```python
from build123d import *

# Parameters (mm, degrees)
SKETCH1_R           = 2
BOSS_EXTRUDE1_DEPTH = 6.35


with BuildPart() as part:
    # Sketch1 → Boss-Extrude1 (new body)
    with BuildSketch(Plane(origin=(0, 0, 0), x_dir=(1, 0, 0), z_dir=(0, 1, 0))):
        with BuildLine():
            Line((12.7, 0), (12.7, 6.35))
            ThreePointArc((12.7, 6.35), (14.559871939, 10.840128061), (19.05, 12.7))
            Line((19.05, 12.7), (39.168815004, 12.7))
            ThreePointArc((39.168815004, 12.7), (45.084999997, 15.87476101), (39.169071524, 19.05))
            Line((39.169071524, 19.05), (12.7, 19.05))
            Line((12.7, 19.05), (10.16, 19.05))
            ThreePointArc((10.16, 19.05), (2.975795103, 16.074204897), (0, 8.89))
            Line((0, 8.89), (0, 0))
            Line((0, 0), (12.7, 0))
        make_face()
        with Locations((41.275, 15.874914922)):
            Circle(SKETCH1_R, mode=Mode.SUBTRACT)
    extrude(amount=BOSS_EXTRUDE1_DEPTH)


solid = part.part
```
The model under review builds one solid part; all positions refer to its coordinate system, in mm. A direction names the side the tool comes from. Round coordinates to 2 decimals unless told otherwise and drop trailing zeros. Loops run counter-clockwise (first coordinate to the right, second up) from the corner with the lowest first, then second, coordinate; pieces in that order, holes last. Notation, with made-up numbers: (7, 53.5) - (56, 53.5) arc R30 cw to (56, 87.5) - close; hole circle Ø4 at (68, 11). An arc over 180 degrees is marked (long way). Use a Markdown table: item, result. Add a question column.
Q1. The part is to be moulded in two halves that separate along X. For faces 1 (the face through (17, 0, -14)), 2 (the face through (14.51, 3.13, -10.79)), 3 (the face through (12.7, 3, -3)), say which applies: pulls with the +X half, pulls with the -X half, needs draft (parallel to the pull), parting line crosses it, or undercut.
Q2. Machinability: for faces 4 (the face through (25, 3, -19.05)), 5 (the face through (39.801, 3.131, -17.227)), 6 (the face through (29, 3, -12.7)), which of the approach directions +Z, -Z, +X, -X, +Y, -Y give a long, thin tool a straight path to every point of the face, cutting with its end or side? Answer none if there is none.
Q3. Add section C-C (y = 2.75). State the section outline as (x, z) points (3 decimals), plus the area to 3 significant figures.
Q4. Add section D-D (x = 26.5). State the section outline as (y, z) points, plus the area to 3 significant figures.
Q5. Insertion check: pin 1 Ø3 at (y, z) = (1, -17.5) entering from -X; pin 2 Ø1.9 at (x, y) = (19.5, 3) entering from -Z; pin 3 Ø1.5 at (x, y) = (17, 4.5) entering from +Z; pin 4 Ø2.5 at (x, z) = (41.28, -15.87) entering from -Y. Each pin has a flat end and moves straight along its axis. Give the tip position at first contact, or say it passes through.
Q6. Add section A-A (z = -17). State the section outline as (x, y) points, plus the area to 3 significant figures.
Q7. For probe 1 along X at (y, z) = (2, -17.25); probe 2 along Z at (x, y) = (33, 3.25); probe 3 along X at (y, z) = (1.5, -3), list the stretches that pass through material, from the lowest coordinate up.
Q8. Add section B-B (x = 42). State the section outline as (y, z) points, plus the area to 3 significant figures.
Worked answers:
| question | item | result |
|---|---|---|
| 1 | face 1 | needs draft |
| 1 | face 2 | undercut |
| 1 | face 3 | pulls with the +X half |
| 2 | face 4 | -Z, -X, +Y, -Y |
| 2 | face 5 | +Y, -Y |
| 2 | face 6 | +Z, +Y, -Y |
| 3 | outline | (0, -8.89) arc R10.16 ccw to (10.16, -19.05) - (39.169, -19.05) arc R3.81 ccw (long way) to (39.169, -12.7) - (19.05, -12.7) arc R6.35 cw to (12.7, -6.35) - (12.7, 0) - (0, 0) - close; hole circle Ø4 at (41.275, -15.875) |
| 3 | area | 422 mm² |
| 4 | outline | (0, -19.05) - (6.35, -19.05) - (6.35, -12.7) - (0, -12.7) - close |
| 4 | area | 40.3 mm² |
| 5 | pin 1 | x = 2.9 |
| 5 | pin 2 | z = -19.05 |
| 5 | pin 3 | z = -12.05 |
| 5 | pin 4 | through |
| 6 | outline | (4.04, 0) - (39.62, 0) - (39.62, 6.35) - (4.04, 6.35) - close; (42.93, 0) - (44.92, 0) - (44.92, 6.35) - (42.93, 6.35) - close |
| 6 | area | 239 mm² |
| 7 | probe 1 | 4.39 to 39.82, 42.73 to 44.83 |
| 7 | probe 2 | -19.05 to -12.7 |
| 7 | probe 3 | 0 to 12.7 |
| 8 | outline | (0, -19.62) - (6.35, -19.62) - (6.35, -17.74) - (0, -17.74) - close; (0, -14.01) - (6.35, -14.01) - (6.35, -12.13) - (0, -12.13) - close |
| 8 | area | 23.8 mm² |
